Solid Edge part; units mm, degrees
sketch "Sketch1" plane through (0, 0, 0) normal (0, 0, 1) x (1, 0, 0)
  line L0 (-32.1803, 100.096) -> (118.4157, 100.096)
  line L1 (118.4157, 100.096) -> (118.4157, -1.5)
  line L2 (118.4157, -1.5) -> (-32.1803, -1.5)
  line L3 (-32.1803, -1.5) -> (-32.1803, 100.096)
  dimension "D1" = 118.4157
  dimension "D2" = 32.1803
extrude "Basiskörper" add sketch "Sketch1" along normal blind 3.798
fillet "Round1" radius 5 4 edges at (118.4157, 100.096, 1.899) (118.4157, -1.5, 1.899) (-32.1803, -1.5, 1.899) (-32.1803, 100.096, 1.899)
sketch "Sketch2" plane through (11.6177, 37.298, 3.798) normal (0, 0, 1) x (1, 0, 0)
  line L0 (-39.5, 58.5) -> (102.5, 58.5)
  line L1 (102.5, 58.5) -> (102.5, -34.5)
  line L2 (102.5, -34.5) -> (-39.5, -34.5)
  line L3 (-39.5, -34.5) -> (-39.5, 58.5)
  dimension "D1" = 39.5
  dimension "D2" = 39.5
extrude "Protrusion1" add sketch "Sketch2" along normal blind 3.798
fillet "Round2" radius 2.202 4 edges at (-27.8823, 95.798, 5.697) (-27.8823, 2.798, 5.697) (114.1177, 2.798, 5.697) (114.1177, 95.798, 5.697)
hole "Hole1" at (111.9457, 4.97, 0) direction (0, 0, 1) diameter 4 end through all counterbore diameter 7 counterbore depth 2.1 start chamfer 0.3 start chamfer angle 45
hole "Hole2" at (111.9457, 93.626, 0) direction (0, 0, 1) diameter 4 end through all counterbore diameter 7 counterbore depth 2.1 start chamfer 0.3 start chamfer angle 45
hole "Hole3" at (-25.7103, 93.626, 0) direction (0, 0, 1) diameter 4 end through all counterbore diameter 7 counterbore depth 2.1 start chamfer 0.3 start chamfer angle 45
hole "Hole4" at (-25.7103, 4.97, 0) direction (0, 0, 1) diameter 4 end through all counterbore diameter 7 counterbore depth 2.1 start chamfer 0.3 start chamfer angle 45
properties material "ASA"
For this review, take the finished solid that the model builds, in its own axes (mm). A direction names the side the tool comes from. Give positions to 0.01 mm unless a question says otherwise; leave off trailing zeros. Loops run counter-clockwise (first coordinate to the right, second up) from the corner with the lowest first, then second, coordinate; pieces in that order, holes last. Notation, with made-up numbers: M 2.25,-40 L 54.25,-40 A8 cw 54.25,-33 Z; hole C 5.5,-26 d3. An arc over 180 degrees is marked long. Put each result on its own line as item: value. Start each with the question number.
(1) Machinability: for faces 5 (the flat face through (44, 2.798, 6)), 6 (the flat face through (49, 1, 3.798)), 7 (the flat face through (-23, 5, 2.1)), 8 (the cylindrical face through (110, 4.5, 4.8)), 9 (the flat face through (-32.18, 49, 2)), which of the approach directions +Z, -Z, +X, -X, +Y, -Y give a long, thin tool a straight path to every point of the face, cutting with its end or side? Answer none if there is none.
(2) Add section A-A, the plane x = 44.5. Write out the cut boundary in (y, z).
(3) The part is to be moulded in two halves that separate along X. For faces 1 (the flat face through (42, 95.798, 6)), 2 (the cylindrical face through (111.79, 90.13, 1.21)), 3 (the cylindrical face through (-29.18, 4.51, 1.21)), 4 (the flat face through (-27.882, 49, 6)), say which applies: +X half, -X half, draft (parallel to the pull), parting line (faces both ways), or undercut.
(4) Add section B-B, the plane z = 5.75. Write out the cut boundary in (x, y), then the cut area to 3 significant figures.
(5) For pin 1 (6.5 mm diameter, centred on x = 111.95, y = 4.97, fed in from -Z); pin 2 (1 mm diameter, centred on x = 97.5, z = 4.5, fed in from +Y); pin 3 (1.9 mm diameter, centred on y = 43, z = 5.5, fed in from -X); pin 4 (3 mm diameter, centred on x = 111.95, y = 4.97, fed in from -Z), all flat-tipped, find the tip position at first contact; note any pin that passes through.
(6) Add section C-C, the plane y = 84. Write out the cut boundary in (x, z).
(7) Wall thickness on L1, parallel to X at y = 4.97, z = 1.15; L2, parallel to X at y = 4.97, z = 5.9; L3, parallel to Y at x = -2.5, z = 5.75: over which ranges is each line inside the solid? List them lowest first.
Result:
1. face 5: +Z, +X, -X, -Y
1. face 6: +Z
1. face 7: -Z
1. face 8: +Z, -Z
1. face 9: +Z, -Z, -X, +Y, -Y
2. outline: M -1.5,0 L 100.1,0 L 100.1,3.8 L 95.8,3.8 L 95.8,7.6 L 2.8,7.6 L 2.8,3.8 L -1.5,3.8 Z
3. face 1: draft
3. face 2: undercut
3. face 3: undercut
3. face 4: -X half
4. outline: M -27.88,5 A2.2 ccw -25.68,2.8 L 111.92,2.8 A2.2 ccw 114.12,5 L 114.12,93.6 A2.2 ccw 111.92,95.8 L -25.68,95.8 A2.2 ccw -27.88,93.6 Z; hole C -25.71,4.97 d4; hole C -25.71,93.63 d4; hole C 111.95,4.97 d4; hole C 111.95,93.63 d4
4. area: 13,200 mm^2
5. pin 1: stops at z = 2.1
5. pin 2: stops at y = 95.8
5. pin 3: stops at x = -27.88
5. pin 4: passes through
6. outline: M -32.18,0 L 118.42,0 L 118.42,3.8 L 114.12,3.8 L 114.12,7.6 L -27.88,7.6 L -27.88,3.8 L -32.18,3.8 Z
7. L1: x = -32.18 to -29.21, -22.21 to 108.45, 115.45 to 118.42
7. L2: x = -27.88 to -27.71, -23.71 to 109.95, 113.95 to 114.12
7. L3: y = 2.8 to 95.8
